from build123d import *

# Parameters (mm, degrees)
SKETCH_W        = 20
SKETCH_H        = 53.5
PAD_DEPTH       = 3
SKETCH001_W     = 20
SKETCH001_H     = 26
PAD001_DEPTH    = 3
FILLET_R        = 1.25
FILLET001_R     = 6
SKETCH002_R     = 2.25
POCKET_DEPTH    = 6
SKETCH003_R     = 3.5
SKETCH003_W     = 8
SKETCH003_H     = 6
POCKET001_DEPTH = 6
FILLET002_R     = 1
POCKET002_DEPTH = 3


with BuildPart() as part:
    # Sketch → Pad (new body)
    with BuildSketch(Plane.XY):
        with Locations((0, 26.75)):
            Rectangle(SKETCH_W, SKETCH_H)
    extrude(amount=PAD_DEPTH)

    # Sketch001 (on Face5 of Pad) → Pad001 (join)
    with BuildSketch(Plane(origin=(0, 0, 0), x_dir=(1, 0, 0), z_dir=(0, 0, -1))):
        with Locations((0, -13)):
            Rectangle(SKETCH001_W, SKETCH001_H)
    extrude(amount=PAD001_DEPTH)

    # Fillet
    fillet_edges = [part.edges().sort_by_distance(p)[0] for p in [
        (0, 26, 0),
        (0, 26, -3),
    ]]
    fillet(fillet_edges, radius=FILLET_R)

    # Fillet001
    fillet001_edges = [part.edges().sort_by_distance(p)[0] for p in [
        (10, 53.5, 1.5),
        (-10, 53.5, 1.5),
    ]]
    fillet(fillet001_edges, radius=FILLET001_R)

    # Sketch002 (on Face12 of Fillet001) → Pocket (cut)
    with BuildSketch(Plane(origin=(0, 0, -3), x_dir=(1, 0, 0), z_dir=(0, 0, -1))):
        with Locations((0, -16)):
            Circle(SKETCH002_R)
    extrude(amount=-POCKET_DEPTH, mode=Mode.SUBTRACT)

    # Sketch003 (on Face8 of Pocket) → Pocket001 (cut)
    with BuildSketch(Plane.XY.offset(3)):
        with Locations((0, 43.5)):
            Circle(SKETCH003_R)
        with Locations((0, 33)):
            Rectangle(SKETCH003_W, SKETCH003_H)
    extrude(amount=-POCKET001_DEPTH, mode=Mode.SUBTRACT)

    # Fillet002
    fillet002_edges = [part.edges().sort_by_distance(p)[0] for p in [
        (-4, 36, 1.5),
        (4, 36, 1.5),
        (4, 30, 1.5),
        (-4, 30, 1.5),
    ]]
    fillet(fillet002_edges, radius=FILLET002_R)

    # Sketch004 (on Face17 of Fillet002) → Pocket002 (cut)
    with BuildSketch(Plane.XY.offset(3)):
        Polygon((2.107328, 19.65), (-2.107328, 19.65), (-4.214657, 16), (-2.107328, 12.35), (2.107328, 12.35), (4.214657, 16), align=None)
    extrude(amount=-POCKET002_DEPTH, mode=Mode.SUBTRACT)


solid = part.part
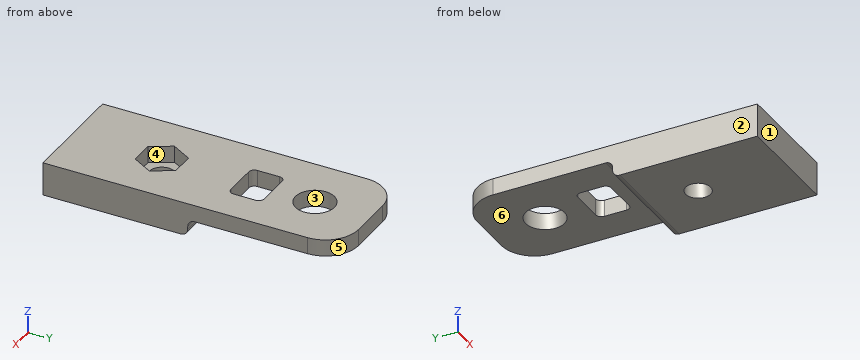
Can you work these out from the model? Positions are in its coordinate system, mm. Face numbers are marked on the shaded views. A direction names the side the tool comes from. Round coordinates to 2 decimals unless told otherwise and drop trailing zeros. Loops run counter-clockwise (first coordinate to the right, second up) from the corner with the lowest first, then second, coordinate; pieces in that order, holes last. Notation, with made-up numbers: (24, 64) - (65, 64) arc R32 cw to (65, 91) - close; hole circle Ø2 at (42, 36). An arc over 180 degrees is marked (long way). Use CSV: the item, a comma, the result in double quotes. Start each with the question number.
1) For the marked faces 5 and 6, which set-ups out of +Z, -Z, +X, -X, +Y, -Y let a thin tool reach every point of the face, with its end or its side?
2) Please list where these lines run through material, in increasing order: probe 1 along Y at (x, z) = (0, 0.7); probe 2 along X at (y, z) = (16, -1.95); probe 3 along Y at (x, z) = (-0.75, 0.95). Write a range as [from, to].
3) If we section it at A-A on y = 43.5: Write out the boundary of the cut face in (x, z).
4) If we section it at C-C on x = 0: Write out the boundary of the cut face in (y, z).
5) For pin 1 Ø1 at (x, z) = (-5, 0.5) entering from +Y; pin 2 Ø1.5 at (y, z) = (35, -1) entering from +X; pin 3 Ø3.5 at (x, y) = (-1, 14) entering from +Z; pin 4 Ø2 at (x, z) = (7, 1.5) entering from +Y, each with a flat end and sliding along its axis, tell me the tip position at first contact or that it passes through.
6) We'd pull the mould along X, two halves only. Please class the marked faces 1, 2, 3 and 4: released by +X, released by -X, zero draft, split by the parting line, or undercut.
7) If we section it at D-D on y = 32.5: Write out the boundary of the cut face in (x, z).
8) If we section it at B-B on z = 1.85: Write out the boundary of the cut face in (x, y), plus the area to 3 significant figures.
Geometry results:
1,face 5,"+Z, -Z, +X, +Y"
1,face 6,"-Z, +X, -X, +Y"
2,probe 1,"y = [0, 12.35], [19.65, 30], [36, 40], [47, 53.5]"
2,probe 2,"x = [-10, -2.25], [2.25, 10]"
2,probe 3,"y = [0, 12.35], [19.65, 30], [36, 40.08], [46.92, 53.5]"
3,outline,"(-10, 0) - (-3.5, 0) - (-3.5, 3) - (-10, 3) - close; (3.5, 0) - (10, 0) - (10, 3) - (3.5, 3) - close"
4,outline,"(0, -3) - (13.75, -3) - (13.75, 0) - (12.35, 0) - (12.35, 3) - (0, 3) - close; (18.25, -3) - (24.75, -3) arc R1.25 ccw to (26, -1.75) - (26, -1.25) arc R1.25 cw to (27.25, 0) - (30, 0) - (30, 3) - (19.65, 3) - (19.65, 0) - (18.25, 0) - close; (36, 0) - (40, 0) - (40, 3) - (36, 3) - close; (47, 0) - (53.5, 0) - (53.5, 3) - (47, 3) - close"
5,pin 1,"stops at y = 53.48"
5,pin 2,"passes through"
5,pin 3,"stops at z = 3"
5,pin 4,"stops at y = 53.16"
6,face 1,"zero draft"
6,face 2,"released by -X"
6,face 3,"undercut"
6,face 4,"undercut"
7,outline,"(-10, 0) - (-4, 0) - (-4, 3) - (-10, 3) - close; (4, 0) - (10, 0) - (10, 3) - (4, 3) - close"
8,outline,"(-10, 0) - (10, 0) - (10, 47.5) arc R6 ccw to (4, 53.5) - (-4, 53.5) arc R6 ccw to (-10, 47.5) - close; hole (-4.21, 16) - (-2.11, 12.35) - (2.11, 12.35) - (4.21, 16) - (2.11, 19.65) - (-2.11, 19.65) - close; hole (-4, 31) arc R1 ccw to (-3, 30) - (3, 30) arc R1 ccw to (4, 31) - (4, 35) arc R1 ccw to (3, 36) - (-3, 36) arc R1 ccw to (-4, 35) - close; hole circle Ø7 at (0, 43.5)"
8,area,"923 mm2"
